from build123d import *

# Parameters (mm, degrees)
F0_R     = 31.75
F1_DEPTH = 12.7
F5_W     = 3.175
F5_H     = 12.7
F8_D     = 4.4958


with BuildPart() as f1:
    # F0 (on Top) → F1 (new body)
    with BuildSketch(Plane.XY):
        Circle(F0_R)
    extrude(amount=F1_DEPTH)

    # F2 (on Front) → F3 (revolve, cut)
    with BuildSketch(Plane.XZ):
        with BuildLine():
            ThreePointArc((0, -3.175), (22.4506403027, 6.1243596973), (31.75, 28.575))
            ThreePointArc((31.75, 28.575), (22.4506403027, 51.0256403027), (0, 60.325))
            Line((0, 60.325), (0, -3.175))
        make_face()
    revolve(axis=Axis((0, 0, 28.575), (0, 0, -1)), mode=Mode.SUBTRACT)

    # F5 (on offset) → F6 (join, up to the next surface of F1)
    with BuildSketch(Plane.YZ.offset(76.2)):
        with Locations((-1.5875, 6.35)):
            Rectangle(F5_W, F5_H)
    extrude(until=Until.NEXT, dir=(-1, 0, 0))

    # F8 (through all)
    with Locations(Plane.XZ.offset(3.175)):
        with Locations((44.45, 6.35), (69.85, 6.35), (57.15, 6.35)):
            Hole(F8_D / 2)


solid = f1.part
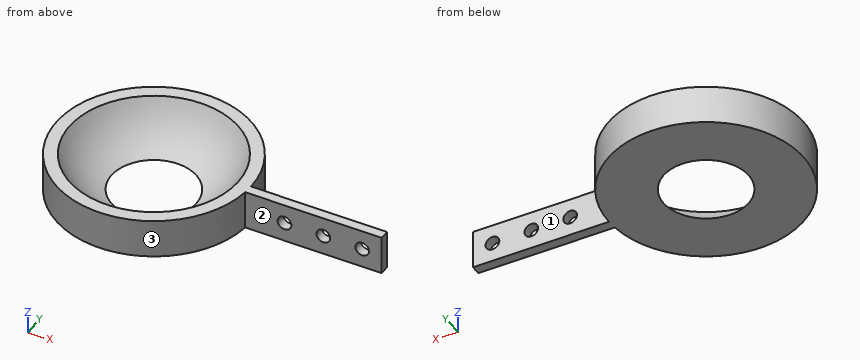
Work out the finished part from the listing and answer in its coordinate system (mm). Face numbers are marked on the shaded views. A direction names the side the tool comes from. Coordinates: 2 decimals unless noted, no trailing zeros. Loops run counter-clockwise (first coordinate to the right, second up) from the corner with the lowest first, then second, coordinate; pieces in that order, holes last. Notation, with made-up numbers: M 18.25,72.25 L 60.25,72.25 A23 ccw 60.25,81.25 Z; hole C 82,24 d5. An arc over 180 degrees is marked long. Answer in a Markdown table with one row per item. Add a question column.
1. Find section C-C, the plane x = -13.5. Write down the section's boundary in (y, z) (3 decimals), then the cut area to 3 significant figures.
2. Find section D-D, the plane y = 20. Write down the section's boundary in (x, z) (3 decimals), then the cut area to 3 significant figures.
3. Consider L1, parallel to Z at x = 44.45, y = -1.35; L2, parallel to Y at x = 41, z = 6 (3 decimals); L3, parallel to Y at x = -5.5, z = 4.5. Determine where each line is inside the solid, lowest interval first.
4. Flat-ended cylindrical pins translate along their axes: P1, Ø6, axis at x = 27, y = -23.5, coming from the -Z side; P2, Ø2, axis at x = -17.5, y = -9.5, coming from the +Z side; P3, Ø1, axis at x = 65, z = 3, coming from the -Y side (3 decimals); P4, Ø6, axis at x = 57.15, z = 6.35, coming from the +Y side. Find the tip coordinate at first contact, or state that the pin passes through.
5. A tool of negligible diameter and unlimited length cuts with its end or side. For the marked faces 1, 2 and 3, from which of +Z, -Z, +X, -X, +Y, -Y can it reach the whole face along a straight path? Write none if from no direction.
6. Find section A-A, the plane z = 6.35. Write down the section's boundary in (x, y) (3 decimals), then the cut area to 3 significant figures.
7. Find section B-B, the plane x = 57.15. Write down the section's boundary in (y, z) (3 decimals).
Reported:
| question | item | result |
|---|---|---|
| 1 | outline | M -28.737,0 L -3.047,0 A28.737 cw -23.954,12.7 L -28.737,12.7 Z; M 3.047,0 L 28.737,0 L 28.737,12.7 L 23.954,12.7 A28.737 cw Z |
| 1 | area | 297 mm^2 |
| 2 | outline | M -24.659,0 L 24.659,0 L 24.659,12.7 L 18.869,12.7 A24.659 cw -18.869,12.7 L -24.659,12.7 Z |
| 2 | area | 396 mm^2 |
| 3 | L1 | z = 0 to 4.1, 8.6 to 12.7 |
| 3 | L2 | y = -3.175 to 0 |
| 3 | L3 | y = -31.27 to -19.96, 19.96 to 31.27 |
| 4 | P1 | passes through |
| 4 | P2 | stops at z = 4.68 |
| 4 | P3 | stops at y = -3.175 |
| 4 | P4 | stops at y = 0 |
| 5 | face 1 | +Z, -Z, +X, +Y |
| 5 | face 2 | +Z, -Z, +X, -Y |
| 5 | face 3 | +Z, -Z |
| 6 | outline | M 31.591,-3.175 L 42.202,-3.175 L 42.202,0 L 31.75,0 A31.75 ccw long Z; M 46.698,-3.175 L 54.902,-3.175 L 54.902,0 L 46.698,0 Z; M 59.398,-3.175 L 67.602,-3.175 L 67.602,0 L 59.398,0 Z; M 72.098,-3.175 L 76.2,-3.175 L 76.2,0 L 72.098,0 Z; hole C 0,0 d45.348 |
| 6 | area | 1,650 mm^2 |
| 7 | outline | M -3.175,0 L 0,0 L 0,4.102 L -3.175,4.102 Z; M -3.175,8.598 L 0,8.598 L 0,12.7 L -3.175,12.7 Z |
